```python
from build123d import *

# Parameters (mm, degrees)
SKETCH2_R           = 2.075
BOSS_EXTRUDE1_DEPTH = 380


with BuildPart() as part:
    # Sketch2 → Boss-Extrude1 (new body)
    with BuildSketch(Plane(origin=(0, 0, 0), x_dir=(0, 0, -1), z_dir=(1, 0, 0))):
        with BuildLine():
            Line((3.125428693, 8.548200862), (3.125428693, 8.203200862))
            Line((3.125428693, 8.203200862), (5.505428693, 8.203200862))
            Line((5.505428693, 8.203200862), (5.505428693, 6.558200862))
            Line((5.505428693, 6.558200862), (2.839571307, 3.903200862))
            Line((2.839571307, 3.903200862), (-2.839571307, 3.903200862))
            Line((-2.839571307, 3.903200862), (-5.505428693, 6.558200862))
            Line((-5.505428693, 6.558200862), (-5.505428693, 8.203200862))
            Line((-5.505428693, 8.203200862), (-3.125428693, 8.203200862))
            Line((-3.125428693, 8.203200862), (-3.125428693, 8.548200862))
            Line((-3.125428693, 8.548200862), (-4.580428693, 10.003200862))
            Line((-4.580428693, 10.003200862), (-9.505428693, 10.003200862))
            ThreePointArc((-9.505428693, 10.003200862), (-9.858982084, 9.856754253), (-10.005428693, 9.503200862))
            Line((-10.005428693, 9.503200862), (-10.005428693, 4.583200862))
            Line((-10.005428693, 4.583200862), (-8.53985696, 3.123200862))
            Line((-8.53985696, 3.123200862), (-8.205428693, 3.123200862))
            Line((-8.205428693, 3.123200862), (-8.205428693, 5.503200862))
            Line((-8.205428693, 5.503200862), (-6.563922349, 5.49537859))
            Line((-6.563922349, 5.49537859), (-3.898064962, 2.84037859))
            Line((-3.898064962, 2.84037859), (-3.898064962, -2.84037859))
            Line((-3.898064962, -2.84037859), (-6.563922349, -5.49537859))
            Line((-6.563922349, -5.49537859), (-8.205428693, -5.503200862))
            Line((-8.205428693, -5.503200862), (-8.205428693, -3.123200862))
            Line((-8.205428693, -3.123200862), (-8.53985696, -3.123200862))
            Line((-8.53985696, -3.123200862), (-10.005428693, -4.583200862))
            Line((-10.005428693, -4.583200862), (-10.005428693, -9.503200862))
            ThreePointArc((-10.005428693, -9.503200862), (-9.858982084, -9.856754253), (-9.505428693, -10.003200862))
            Line((-9.505428693, -10.003200862), (-4.580428693, -10.003200862))
            Line((-4.580428693, -10.003200862), (-3.125428693, -8.548200862))
            Line((-3.125428693, -8.548200862), (-3.125428693, -8.203200862))
            Line((-3.125428693, -8.203200862), (-5.505428693, -8.203200862))
            Line((-5.505428693, -8.203200862), (-5.505428693, -6.558200862))
            Line((-5.505428693, -6.558200862), (-2.839571307, -3.903200862))
            Line((-2.839571307, -3.903200862), (2.839571307, -3.903200862))
            Line((2.839571307, -3.903200862), (5.505428693, -6.558200862))
            Line((5.505428693, -6.558200862), (5.505428693, -8.203200862))
            Line((5.505428693, -8.203200862), (3.125428693, -8.203200862))
            Line((3.125428693, -8.203200862), (3.125428693, -8.548200862))
            Line((3.125428693, -8.548200862), (4.580428693, -10.003200862))
            Line((4.580428693, -10.003200862), (15.430428693, -10.003200862))
            Line((15.430428693, -10.003200862), (16.885428693, -8.548200862))
            Line((16.885428693, -8.548200862), (16.885428693, -8.203200862))
            Line((16.885428693, -8.203200862), (14.505428693, -8.203200862))
            Line((14.505428693, -8.203200862), (14.505428693, -6.558200862))
            Line((14.505428693, -6.558200862), (17.17128608, -3.903200862))
            Line((17.17128608, -3.903200862), (22.850428693, -3.903200862))
            Line((22.850428693, -3.903200862), (25.51628608, -6.558200862))
            Line((25.51628608, -6.558200862), (25.51628608, -8.203200862))
            Line((25.51628608, -8.203200862), (23.13628608, -8.203200862))
            Line((23.13628608, -8.203200862), (23.13628608, -8.548200862))
            Line((23.13628608, -8.548200862), (24.59128608, -10.003200862))
            Line((24.59128608, -10.003200862), (29.51628608, -10.003200862))
            ThreePointArc((29.51628608, -10.003200862), (29.869839471, -9.856754253), (30.01628608, -9.503200862))
            Line((30.01628608, -9.503200862), (30.01628608, -4.583200862))
            Line((30.01628608, -4.583200862), (28.550714346, -3.123200862))
            Line((28.550714346, -3.123200862), (28.21628608, -3.123200862))
            Line((28.21628608, -3.123200862), (28.21628608, -5.503200862))
            Line((28.21628608, -5.503200862), (26.574779736, -5.49537859))
            Line((26.574779736, -5.49537859), (23.908922349, -2.84037859))
            Line((23.908922349, -2.84037859), (23.908922349, 2.84037859))
            Line((23.908922349, 2.84037859), (26.574779736, 5.49537859))
            Line((26.574779736, 5.49537859), (28.21628608, 5.503200862))
            Line((28.21628608, 5.503200862), (28.21628608, 3.123200862))
            Line((28.21628608, 3.123200862), (28.550714346, 3.123200862))
            Line((28.550714346, 3.123200862), (30.01628608, 4.583200862))
            Line((30.01628608, 4.583200862), (30.01628608, 9.503200862))
            ThreePointArc((30.01628608, 9.503200862), (29.869839471, 9.856754253), (29.51628608, 10.003200862))
            Line((29.51628608, 10.003200862), (24.59128608, 10.003200862))
            Line((24.59128608, 10.003200862), (23.13628608, 8.548200862))
            Line((23.13628608, 8.548200862), (23.13628608, 8.203200862))
            Line((23.13628608, 8.203200862), (25.51628608, 8.203200862))
            Line((25.51628608, 8.203200862), (25.51628608, 6.558200862))
            Line((25.51628608, 6.558200862), (22.850428693, 3.903200862))
            Line((22.850428693, 3.903200862), (17.17128608, 3.903200862))
            Line((17.17128608, 3.903200862), (14.505428693, 6.558200862))
            Line((14.505428693, 6.558200862), (14.505428693, 8.203200862))
            Line((14.505428693, 8.203200862), (16.885428693, 8.203200862))
            Line((16.885428693, 8.203200862), (16.885428693, 8.548200862))
            Line((16.885428693, 8.548200862), (15.430428693, 10.003200862))
            Line((15.430428693, 10.003200862), (4.580428693, 10.003200862))
            Line((4.580428693, 10.003200862), (3.125428693, 8.548200862))
        make_face()
        with Locations((0.003681866, 0)):
            Circle(SKETCH2_R, mode=Mode.SUBTRACT)
        with Locations((20.007175521, 0)):
            Circle(SKETCH2_R, mode=Mode.SUBTRACT)
        Polygon((3.898064962, 2.84037859), (3.898064962, -2.84037859), (6.90134296, -5.83142497), (6.90134296, -8.203200862), (13.109514426, -8.203200862), (13.109514426, -5.83142497), (16.112792425, -2.84037859), (16.112792425, 2.84037859), (13.109514426, 5.83142497), (13.109514426, 8.203200862), (6.90134296, 8.203200862), (6.90134296, 5.83142497), align=None, mode=Mode.SUBTRACT)
    extrude(amount=BOSS_EXTRUDE1_DEPTH)


solid = part.part
```
Geometry check sheet. Reference: the model listing, model coordinates, mm. A direction names the side the tool comes from. Coordinates: 2 decimals unless noted, no trailing zeros.
Item 1: Sectioned sample at A-A, the plane x = 129. Count the separate pieces of the cut face and the enclosed holes in it, then the cut area to 3 significant figures.
Item 2: Go/stop test with a flat-tipped pin: pin 1 Ø1.5 at (x, y) = (253.5, 0.5) entering from +Z. Record where the tip stops, or that it passes through.
Item 3: Release check for a two-part mould opening along Y. For faces 3 (the face through (380, 5, -5)), 4 (the face through (187, -10.003, -10)), 5 (the face through (187, -8.203, -10)) record: released by +Y, released by -Y, zero draft, split by the parting line, or undercut.
Item 4: Access from +Z, -Z, +X, -X, +Y, -Y to the whole of each face (thin tool, end or side, straight path). Record for faces 1 (the face through (187, 10.003, -10)), 2 (the face through (187, 8.203, -10)).
Item 5: Thickness scan on line 1 (Z direction, x = 23.5, y = 6.75); line 2 (Y direction, x = 62, z = -11); line 3 (Y direction, x = 186, z = 5). Record the ranges inside material, lowest first.
Check result:
1. separate pieces: 1
1. enclosed holes: 3
1. area: 298 mm2
2. pin 1: stops at z = 3.9
3. face 3: zero draft
3. face 4: released by -Y
3. face 5: undercut
4. face 1: +Z, -Z, +X, -X, +Y
4. face 2: +X, -X
5. line 1: z = -30.02 to -25.52, -14.51 to -13.11, -6.9 to -5.51, 5.51 to 10.01
5. line 2: y = -10 to -8.2, 8.2 to 10
5. line 3: y = -10 to -8.2, -6.05 to -3.94, 3.94 to 6.05, 8.2 to 10
